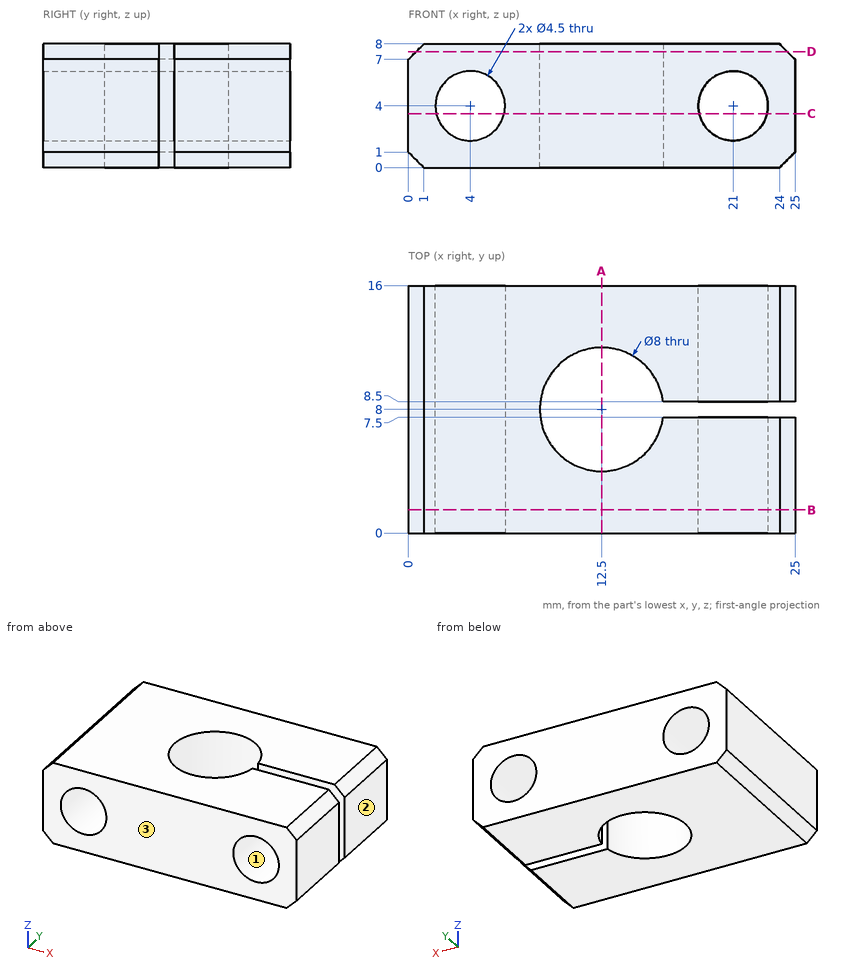
Print and shaded views of the part. All mm, measured from the part's lowest x, y and z. Coordinates: 2 decimals unless noted, no trailing zeros. Write each loop counter-clockwise with the first axis right and the second up, starting at its lowest first coordinate (ties: lowest second). Pieces come first, ordered by that corner, then holes. Notation, with made-up numbers: M 68,85.5 L 96,85.5 A13 ccw 96,98.5 Z; hole C 78,69 d5. An arc over 180 degrees is marked long. Return JSON: item names as keys, results as strings.
1. Saw through at B-B, the plane y = 1.5. Write the cut outline in (x, z), then the cut area to 3 significant figures.
Determined:
{"outline": "M 0,1 L 1,0 L 24,0 L 25,1 L 25,7 L 24,8 L 1,8 L 0,7 Z; hole C 4,4 d4.5; hole C 21,4 d4.5", "area": "166 mm²"}
2. Saw through at D-D, the plane z = 7.5. Write the cut outline in (x, y), then the cut area to 3 significant figures.
Determined:
{"outline": "M 0.5,0 L 24.5,0 L 24.5,7.5 L 16.47,7.5 A4 cw long 16.47,8.5 L 24.5,8.5 L 24.5,16 L 0.5,16 Z", "area": "326 mm²"}
3. Flat gauge pin, fed straight in: pin 1 Ø3 at (x, z) = (22.5, 5.5) entering from -Y. Where does the tip first touch, or does it go through?
Determined:
{"pin 1": "y = 0"}
4. Pull direction X, two halves, no side cores. Call the marked faces 1, 2 and 3: pulls with the +X half, pulls with the -X half, needs draft (parallel to the pull), parting line crosses it, or undercut.
Determined:
{"face 1": "undercut", "face 2": "pulls with the +X half", "face 3": "needs draft"}
5. Saw through at C-C, the plane z = 3.5. Write the cut outline in (x, y), then the cut area to 3 significant figures.
Determined:
{"outline": "M 0,0 L 1.81,0 L 1.81,16 L 0,16 Z; M 6.19,0 L 18.81,0 L 18.81,7.5 L 16.47,7.5 A4 cw long 16.47,8.5 L 18.81,8.5 L 18.81,16 L 6.19,16 Z; M 23.19,0 L 25,0 L 25,7.5 L 23.19,7.5 Z; M 23.19,8.5 L 25,8.5 L 25,16 L 23.19,16 Z", "area": "205 mm²"}
6. Probe L1, parallel to Z at x = 4, y = 11; L2, parallel to Y at x = 24, z = 3.5; L3, parallel to X at y = 9.5, z = 3.25. List the from-to ranges inside material, lowest first.
Determined:
{"L1": "0 to 1.75, 6.25 to 8", "L2": "0 to 7.5, 8.5 to 16", "L3": "0 to 1.88, 6.12 to 8.79, 16.21 to 18.88, 23.12 to 25"}
7. Saw through at A-A, the plane x = 12.5. Write the cut outline in (y, z).
Determined:
{"outline": "M 0,0 L 4,0 L 4,8 L 0,8 Z; M 12,0 L 16,0 L 16,8 L 12,8 Z"}
